Part model, mm, in its own coordinate system. Face numbers are marked on the shaded views. Round coordinates to 2 decimals unless told otherwise and drop trailing zeros. Write each loop counter-clockwise with the first axis right and the second up, starting at its lowest first coordinate (ties: lowest second). Pieces come first, ordered by that corner, then holes. Notation, with made-up numbers: (20.25, -29.5) -> (78.25, -29.5) arc R25 cw to (78.25, 3.5) -> close; hole circle Ø10 at (-2, 86.5). An arc over 180 degrees is marked (long way). Return JSON: item names as keys, results as strings. Group by question number.
(1) Saw through at B-B (x = 0). List the corners of the cut face in (y, z) (3 decimals).
(2) Saw through at D-D (z = 725.5). List the corners of the cut face in (x, y) (3 decimals).
(3) Mould opens along Y. For the marked faces 1 and 2 say: +Y half, -Y half, draft (parallel to the pull), parting line (faces both ways), or undercut.
(4) Saw through at A-A (y = 0). List the corners of the cut face in (x, z) (3 decimals).
(5) Drill centre lines: L1, parallel to Z at x = 0, y = -150.85; L2, parallel to Y at x = 67.5, z = 922; L3, parallel to Y at x = 89, z = 61. Where is each one in solid material? Low to high. Write a range as from..to.
(6) Drop flat-ended pins along their axis: pin 1 Ø10 at (x, z) = (80, 891.5) entering from +Y; pin 2 Ø8 at (y, z) = (115, 482.5) entering from -X; pin 3 Ø4 at (y, z) = (84, 325) entering from -X. Give the stop position or say it passes through.
from build123d import *

# Parameters (mm, degrees)
SKETCH1_R               = 152.4
BOSS_EXTRUDE1_DEPTH     = 1016
SKETCH2_R               = 149.225
CUT_EXTRUDE1_DEPTH      = 1016
SKETCH4_R               = 19.05
CUT_EXTRUDE3_DEPTH      = 441.96
CUT_EXTRUDE3_DEPTH_BACK = 459.754024061


with BuildPart() as part:
    # Sketch1 → Boss-Extrude1 (new body)
    with BuildSketch(Plane.XY):
        Circle(SKETCH1_R)
    extrude(amount=BOSS_EXTRUDE1_DEPTH)

    # Sketch2 → Cut-Extrude1 (cut)
    with BuildSketch(Plane.XY.offset(1016)):
        Circle(SKETCH2_R)
    extrude(amount=-CUT_EXTRUDE1_DEPTH, mode=Mode.SUBTRACT)

    # Sketch4 → Cut-Extrude3 (cut, two sides)
    with BuildSketch(Plane(origin=(0, 0, 0), x_dir=(1, 0, 0), z_dir=(0, 1, 0))) as cut_extrude3_sk:
        with Locations((0, -508)):
            Circle(SKETCH4_R)
    extrude(amount=CUT_EXTRUDE3_DEPTH, mode=Mode.SUBTRACT)
    extrude(cut_extrude3_sk.sketch, amount=-CUT_EXTRUDE3_DEPTH_BACK, mode=Mode.SUBTRACT)


solid = part.part
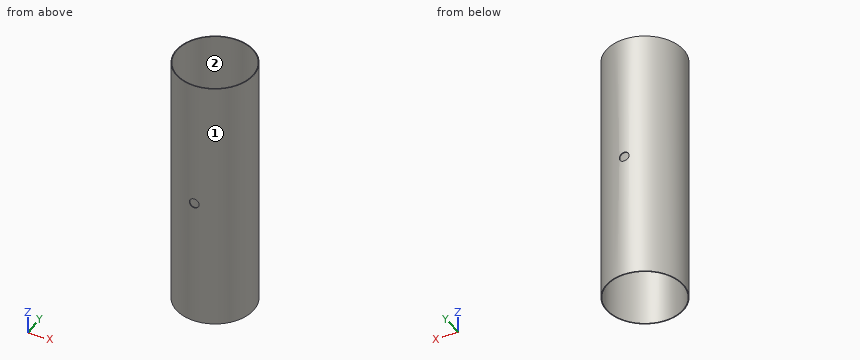
Computed values:
{
 "1": {"outline": "(-152.4, 0) -> (-149.225, 0) -> (-149.225, 488.95) -> (-152.4, 488.95) -> close; (-152.4, 527.05) -> (-149.225, 527.05) -> (-149.225, 1016) -> (-152.4, 1016) -> close; (149.225, 0) -> (152.4, 0) -> (152.4, 488.95) -> (149.225, 488.95) -> close; (149.225, 527.05) -> (152.4, 527.05) -> (152.4, 1016) -> (149.225, 1016) -> close"},
 "2": {"outline": "circle Ø304.8 at (0, 0); hole circle Ø298.45 at (0, 0)"},
 "3": {"face 1": "parting line", "face 2": "undercut"},
 "4": {"outline": "(-152.4, 0) -> (-149.225, 0) -> (-149.225, 1016) -> (-152.4, 1016) -> close; (149.225, 0) -> (152.4, 0) -> (152.4, 1016) -> (149.225, 1016) -> close"},
 "5": {"L1": "0..488.95, 527.05..1016", "L2": "-136.64..-133.09, 133.09..136.64", "L3": "-123.71..-119.78, 119.78..123.71"},
 "6": {"pin 1": "y = 132.67", "pin 2": "x = -104.43", "pin 3": "x = -128.46"}
}
